Verification items for this drawing (mm, ordinates from the low corner). A direction names the side the tool comes from. Round coordinates to 2 decimals unless told otherwise and drop trailing zeros. Loops run counter-clockwise (first coordinate to the right, second up) from the corner with the lowest first, then second, coordinate; pieces in that order, holes last. Notation, with made-up numbers: (11, 60) - (56, 60) arc R23 cw to (56, 68) - close; hole circle Ø5 at (73.5, 44). An arc over 180 degrees is marked (long way). Write item = value, one per line.
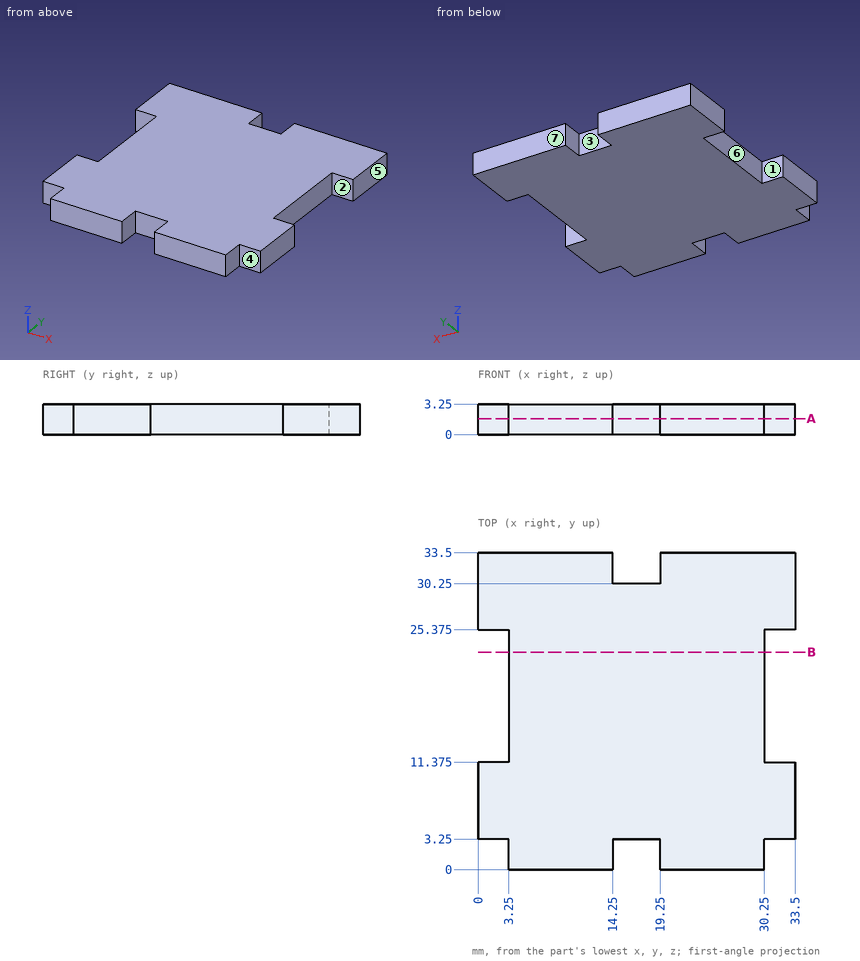
(1) Scan lines: L1, parallel to Y at x = 32, z = 2.75 (3 decimals); L2, parallel to X at y = 31.5, z = 2.75; L3, parallel to X at y = 14, z = 1.05. Record each from-to range of solid material in increasing order. Write a range as [from, to].
Answers follow:
L1 = [3.25, 11.375], [25.375, 33.5]
L2 = [0, 14.25], [19.25, 33.5]
L3 = [3.25, 30.25]
(2) Mould release check, pull along Y, two halves, no side actions. Record for the marked faces 5, 6 and 7: pulls with the +Y half, pulls with the -Y half, needs draft (parallel to the pull), parting line crosses it, or undercut.
Answers follow:
face_5 = needs draft
face_6 = undercut
face_7 = pulls with the +Y half
(3) Section check A-A (z = 1.7). Enter the section's corners in (x, y) (3 decimals), then the cut area to 3 significant figures.
Answers follow:
outline = (0, 3.25) - (3.25, 3.25) - (3.25, 0) - (14.25, 0) - (14.25, 3.25) - (19.25, 3.25) - (19.25, 0) - (30.25, 0) - (30.25, 3.25) - (33.5, 3.25) - (33.5, 11.375) - (30.25, 11.375) - (30.25, 25.375) - (33.5, 25.375) - (33.5, 33.5) - (19.25, 33.5) - (19.25, 30.25) - (14.25, 30.25) - (14.25, 33.5) - (0, 33.5) - (0, 25.375) - (3.25, 25.375) - (3.25, 11.375) - (0, 11.375) - close
area = 978 mm²
(4) Set-up check for the marked faces 1, 2, 3 and 4: record each of +Z, -Z, +X, -X, +Y, -Y from which the full face is reachable in a straight line by a thin tool's end or side.
Answers follow:
face_1 = +Z, -Z, -X
face_2 = +Z, -Z, +X
face_3 = +Z, -Z, +Y
face_4 = +Z, -Z, +X, -Y
(5) Gauge pin test, flat ends, axial feed: pin 1 (1 mm diameter, centred on y = 18, z = 1, fed in from +X); pin 2 (1 mm diameter, centred on x = 31.5, z = 1, fed in from -Y). Record the tip position at first contact, or that the pin passes through.
Answers follow:
pin_1 = 30.25
pin_2 = 3.25
(6) Section check B-B (y = 23). Enter the section's corners in (x, z), then the cut area to 4 significant figures.
Answers follow:
outline = (3.25, 0) - (30.25, 0) - (30.25, 3.25) - (3.25, 3.25) - close
area = 87.75 mm²
